from build123d import *

# Parameters (mm, degrees)
F0_R     = 60
F1_DEPTH = 120
F1_TAPER = 5
F2_T     = -2
F4_R     = 19.3884606064
F5_DEPTH = 120
F5_TAPER = 7


with BuildPart() as f1:
    # F0 (on Top) → F1 (new body)
    with BuildSketch(Plane.XY):
        Circle(F0_R)
    extrude(amount=F1_DEPTH, taper=F1_TAPER)

    # F2
    f2_openings = [f1.faces().sort_by_distance(p)[0] for p in [
        (0, 0, 120),
    ]]
    offset(amount=F2_T, openings=f2_openings)

    # F4 (on offset) → F5 (join, through all)
    with BuildSketch(Plane.XY.offset(120)):
        with Locations((0, -61.8580617011)):
            Circle(F4_R)
    extrude(amount=-F5_DEPTH, taper=F5_TAPER)


solid = f1.part
Read the model definition and answer for the solid it produces. Units are mm, in the model's axes. A direction names the side the tool comes from. Coordinates: 2 decimals unless noted, no trailing zeros. Write each loop counter-clockwise with the first axis right and the second up, starting at its lowest first coordinate (ties: lowest second). Pieces come first, ordered by that corner, then holes. Notation, with made-up numbers: (33, -28) - (78, -28) arc R18 ccw to (78, 0) - close; hole circle Ø10 at (-9.5, -1). An arc over 180 degrees is marked (long way). One line per question, with ' | ' between items.
Q1. Find section C-C, the plane z = 50. Write down the section's boundary in (x, y).
Result set:
outline: (-8.33, -55) arc R10.79 ccw (long way) to (8.33, -55) arc R55.63 ccw (long way) to start; hole (-6.48, -53.23) arc R10.79 cw to (6.48, -53.23) arc R53.62 ccw (long way) to start
Q2. Find section B-B, the plane x = 0. Write down the section's boundary in (y, z).
Result set:
outline: (-81.25, 120) - (-66.51, 0) - (60, 0) - (49.5, 120) - (47.49, 120) - (57.82, 2) - (-56.96, 2) - (-42.47, 120) - close
Q3. For faces 1 (the flat face through (-1, -2, 0)), 2 (the conical face through (0.112, -49.816, 60.174)), determine the directions among +Z, -Z, +X, -X, +Y, -Y from which every point of the face is accessible in a straight line to the end or side of a thin tool.
Result set:
face 1: -Z, +X, -X, +Y, -Y | face 2: none
Q4. Determine the mould class of faces 3 (the conical face through (-0.4, -73.77, 59.16)), 4 (the flat face through (0, -45, 120)) for opening direction Y: +Y half, -Y half, draft (parallel to the pull), parting line (faces both ways), or undercut.
Result set:
face 3: undercut | face 4: draft
Q5. Find section A-A, the plane z = 102. Write down the section's boundary in (x, y), plus the area to 3 significant figures.
Result set:
outline: (-12.07, -49.63) arc R17.18 ccw (long way) to (12.07, -49.63) arc R51.08 ccw (long way) to start; hole (-10.16, -48.01) arc R17.18 cw to (10.16, -48.01) arc R49.07 ccw (long way) to start | area: 1,510 mm^2
Q6. Each of these flat-tipped pins is pushed along its axis until it touches: P1, Ø2, axis at x = -19, y = 4, coming from the -Z side; P2, Ø3, axis at x = -44, z = 29, coming from the +Y side; P3, Ø5, axis at x = 25, z = 24, coming from the -Y side; P4, Ø8, axis at y = -13, z = 74, coming from the +X side. Where does it stop, or does it pass through?
Result set:
P1: z = 0 | P2: y = 38.69 | P3: y = -53.38 | P4: x = 52.85
Q7. Consider L1, parallel to Z at x = -7.5, y = 37; L2, parallel to Y at x = 30, z = 10; L3, parallel to Y at x = 34, z = 53. Determine where each line is inside the solid, lowest interval first. Write a range as [from, to].
Result set:
L1: [0, 2] | L2: [-50.95, -48.6], [48.6, 50.95] | L3: [-43.69, -41.12], [41.12, 43.69]
